Could you check a few things on this model? Use its own coordinates, in mm. Coordinates: 2 decimals unless noted, no trailing zeros. Order: outer loops, then holes, each group sorted by start corner. A loop starts at its lowest first (then second) coordinate and runs counter-clockwise, first axis right, second up. Notation, with made-up numbers: (48, 84.25) -> (79, 84.25) arc R19 cw to (79, 113.25) -> close; hole circle Ø10 at (-18, 63.5). An arc over 180 degrees is marked (long way). Use a Markdown table: item, result. Add a question column.
1) If we section it at A-A (z = 1.7): Write out the boundary of the cut face in (x, y), plus the area to 3 significant figures.
2) Will this pin go through, and if not, where does the flat tip stop? pin 1 Ø2.5 at (x, y) = (57.57, 85.67) entering from -Z.
3) If I drill on L1, parallel to X at y = 79.5, z = 2.2; L2, parallel to X at y = 78.5, z = 0.95; L3, parallel to X at y = 87, z = 2.3, over which ranges is the centre line in solid material (lowest first)? Write a range as [from, to].
```python
from build123d import *

# Parameters (mm, degrees)
BOSS_EXTRUDE1_DEPTH  = 4
M3_CLEARANCE_HOLE1_D = 3.2
M3_CLEARANCE_HOLE2_D = 3.4


with BuildPart() as part:
    # Sketch1 → Boss-Extrude1 (new body)
    with BuildSketch(Plane.XY):
        with BuildLine():
            Line((59.571068699, 89.405091171), (-178.928931301, 89.405091171))
            ThreePointArc((-178.928931301, 89.405091171), (-181.050251645, 88.526411514), (-181.928931301, 86.405091171))
            Line((-181.928931301, 86.405091171), (-181.928931301, 75.539261619))
            Line((-181.928931301, 75.539261619), (62.571068699, 75.539261619))
            Line((62.571068699, 75.539261619), (62.571068699, 86.405091171))
            ThreePointArc((62.571068699, 86.405091171), (61.692389042, 88.526411514), (59.571068699, 89.405091171))
        make_face()
    extrude(amount=BOSS_EXTRUDE1_DEPTH)

    # M3 Clearance Hole1 (through all)
    with Locations(Plane.XY.offset(4)):
        with Locations((-176.928931301, 85.672841171), (-176.928931301, 79.172841171), (-161.428931301, 79.172841171), (47.571068699, 79.172841171), (57.571068699, 79.172841171), (57.571068699, 85.672841171)):
            Hole(M3_CLEARANCE_HOLE1_D / 2)

    # M3 Clearance Hole2 (through all)
    with Locations(Plane(origin=(0, 0, 0), x_dir=(-1, 0, 0), z_dir=(0, 0, -1))):
        with Locations((120.8322952, 78.075091171)):
            Hole(M3_CLEARANCE_HOLE2_D / 2)


solid = part.part
```
Answer sheet:
| question | item | result |
|---|---|---|
| 1 | outline | (-181.93, 75.54) -> (62.57, 75.54) -> (62.57, 86.41) arc R3 ccw to (59.57, 89.41) -> (-178.93, 89.41) arc R3 ccw to (-181.93, 86.41) -> close; hole circle Ø3.2 at (-176.93, 79.17); hole circle Ø3.2 at (-176.93, 85.67); hole circle Ø3.2 at (-161.43, 79.17); hole circle Ø3.4 at (-120.83, 78.08); hole circle Ø3.2 at (47.57, 79.17); hole circle Ø3.2 at (57.57, 79.17); hole circle Ø3.2 at (57.57, 85.67) |
| 1 | area | 3,330 mm2 |
| 2 | pin 1 | through |
| 3 | L1 | [-181.93, -178.5], [-175.36, -163], [-159.86, -121.76], [-119.91, 46], [49.14, 56], [59.14, 62.57] |
| 3 | L2 | [-181.93, -178.38], [-175.48, -162.88], [-159.98, -122.48], [-119.19, 46.12], [49.02, 56.12], [59.02, 62.57] |
| 3 | L3 | [-181.87, -177.82], [-176.04, 56.68], [58.46, 62.51] |
